from build123d import *

# Parameters (mm, degrees)
SKETCH5_R          = 4.7625
CUT_EXTRUDE2_DEPTH = 239.324208658


with BuildPart() as part:
    # Sketch1 → Revolve1 (revolve)
    with BuildSketch(Plane.XY, mode=Mode.PRIVATE) as revolve1_sk:
        Polygon((66.717724762, 49.046294838), (66.717724762, 251.12966618), (47.613204362, 251.12966618), (51.009563545, 49.046294838), align=None)
    revolve(revolve1_sk.sketch.rotate(Axis((66.717724762, 49.046294838, 0), (0, 1, 0)), 270), axis=Axis((66.717724762, 49.046294838, 0), (0, 1, 0)))

    # Sketch4 → Revolve3 (revolve)
    with BuildSketch(Plane.XY):
        with BuildLine():
            Line((66.717724762, 251.12966618), (66.717724762, 270.557968954))
            ThreePointArc((66.717724762, 270.557968954), (53.093833538, 264.847592826), (47.613204362, 251.12966618))
            Line((47.613204362, 251.12966618), (66.717724762, 251.12966618))
        make_face()
    revolve(axis=Axis((66.717724762, 251.12966618, 0), (0, 1, 0)))

    # Sketch5 → Cut-Extrude2 (cut, through all)
    with BuildSketch(Plane.XZ.offset(-49.046294838)):
        with Locations(Location((66.717724762, 0, 0), (0, 0, 270))):
            Circle(SKETCH5_R)
    extrude(amount=-CUT_EXTRUDE2_DEPTH, mode=Mode.SUBTRACT)


solid = part.part
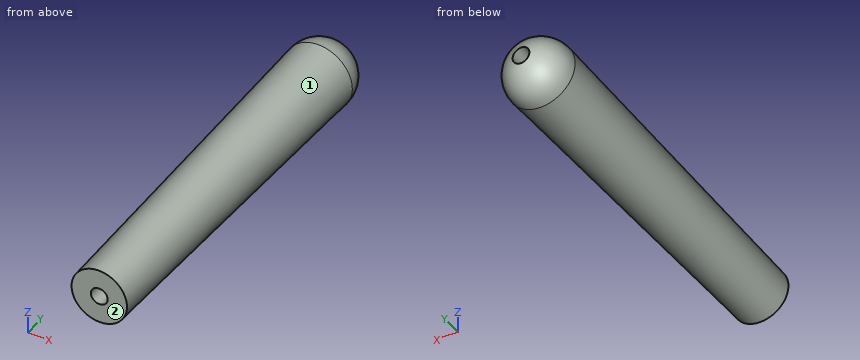
The listing builds one solid part. Answer for the finished solid, in the listing's coordinates (mm). Face numbers are marked on the shaded views. A direction names the side the tool comes from. Coordinates: 2 decimals unless noted, no trailing zeros. Loops run counter-clockwise (first coordinate to the right, second up) from the corner with the lowest first, then second, coordinate; pieces in that order, holes last.
1) Find section B-B on y = 156.5. Write down the section's boundary in (x, z) (1 decimal).
2) Flat-ended cylindrical pins translate along their axes: pin 1 Ø3 at (y, z) = (184.5, 11) entering from -X; pin 2 Ø5 at (x, y) = (68.5, 73.5) entering from +Z; pin 3 Ø1.5 at (y, z) = (127.5, -13.5) entering from -X. Find the tip coordinate at first contact, or state that the pin passes through.
3) Find the intervals of material crossed by L1, parallel to X at y = 135.5, z = 0; L2, parallel to X at y = 126.5, z = 3.5; L3, parallel to Z at x = 65, y = 96.5, in increasing order.
4) A tool of negligible diameter and unlimited length cuts with its end or side. For the marked faces 1 and 2, from which of +Z, -Z, +X, -X, +Y, -Y can it reach the whole face along a straight path? Write none if from no direction.
5) Find section A-A on y = 73. Write down the section's boundary in (x, z) (1 decimal).
Values:
1. outline: circle Ø35 at (66.7, 0); hole circle Ø9.5 at (66.7, 0)
2. pin 1: stops at x = 51.45
2. pin 2: stops at z = 16.15
2. pin 3: stops at x = 55.43
3. L1: x = 49.56 to 61.96, 71.48 to 83.88
3. L2: x = 50.07 to 63.49, 69.95 to 83.36
3. L3: z = -16.42 to -4.44, 4.44 to 16.42
4. face 1: -Y
4. face 2: +Z, -Z, +X, -X, -Y
5. outline: circle Ø32.2 at (66.7, 0); hole circle Ø9.5 at (66.7, 0)
